Autodesk Inventor part; units mm, degrees
ref_plane "YZ Plane" through (0, 0, 0) normal (1, 0, 0) x (0, 1, 0)
ref_plane "XZ Plane" through (0, 0, 0) normal (0, 1, 0) x (-1, 0, 0)
ref_plane "XY Plane" through (0, 0, 0) normal (0, 0, 1) x (1, 0, 0)
sketch "草圖1" plane through (0, 0, 0) normal (0, 1, 0) x (-1, 0, 0)
  line L0 (14, 14) -> (-14, 14)
  line L1 (-14, 14) -> (-14, -14)
  line L2 (-14, -14) -> (14, -14)
  line L3 (14, -14) -> (14, 14)
  line L4 (14, 14) -> (-14, -14) construction
  line L5 (-14, 14) -> (14, -14) construction
  point P0 (0, 0)
  dimension "d0" = 28
  dimension "d1" = 28
extrude "擠出1" add sketch "草圖1" along normal blind 36
sketch "草圖2" plane through (0, 36, 0) normal (0, 1, 0) x (1, 0, 0)
  circle A0 centre (0, 0) radius 14
extrude "擠出2" add sketch "草圖2" along normal blind 28
sketch "草圖3" plane through (0, 64, 0) normal (0, 1, 0) x (1, 0, 0)
  circle A0 centre (0, 0) radius 8.5
  dimension "d6" = 17
extrude "擠出3" add sketch "草圖3" along normal blind 2
sketch "草圖4" plane through (0, 66, 0) normal (0, 1, 0) x (1, 0, 0)
  circle A0 centre (0, 0) radius 3
  dimension "d9" = 6
extrude "擠出4" add sketch "草圖4" along normal blind 17.5
sketch "草圖5" plane through (0, 83.5, 0) normal (0, 1, 0) x (1, 0, 0)
  circle A0 centre (0, 0) radius 3
  line L0 (-2.5, -1.6583) -> (-2.5, 1.6583)
  point P0 (3, 0)
  dimension "d13" = 5.5
extrude "擠出5" cut sketch "草圖5" against normal blind 15 contours L0 A0 picked at (-2.6056, 0.3442)
sketch "草圖6" plane through (0, 64, 0) normal (0, 1, 0) x (1, 0, 0)
  circle A0 centre (0, 0) radius 11 construction
  line L0 (0, 0) -> (0, 11) construction
  circle A1 centre (0, 0) radius 14
  line L1 (14, 14) -> (0, 14)
  line L2 (-14, -14) -> (0, -14)
  line L3 (14, 14) -> (-14, -14) construction
  circle A2 centre (7.7782, 7.7782) radius 1.5
  circle A3 centre (-7.7782, 7.7782) radius 1.5
  circle A4 centre (-7.7782, -7.7782) radius 1.5
  circle A5 centre (7.7782, -7.7782) radius 1.5
  dimension "d16" = 22
  dimension "d24" = 3
  dimension "d27" = 360
extrude "擠出6" cut sketch "草圖6" against normal blind 10 contours A2 | A3 | A4 | A5
properties part number "28stepper27"
Design review of the part built by this model. Coordinates are the model's own, in mm. A direction names the side the tool comes from. Give positions to 0.01 mm unless a question says otherwise; leave off trailing zeros. Order: outer loops, then holes, each group sorted by start corner. A loop starts at its lowest first (then second) coordinate and runs counter-clockwise, first axis right, second up. Notation, with made-up numbers: (23.25, -4.5) - (51.25, -4.5) arc R12 cw to (51.25, 6.5) - close; hole circle Ø10 at (79.25, 8.25). An arc over 180 degrees is marked (long way). Write item = value, one per line. Start each with the question number.
Q1. We need section A-A on x = 11. State the section outline as (y, z) points.
Q2. To check wall thickness, follow L1, parallel to Y at x = 6.75, z = -1; L2, parallel to Z at x = 8.25, y = 56; L3, parallel to Y at x = 0, z = 12.75. State the ranges of each line that lie inside material, in increasing order. Write a range as from..to.
Q3. Clearance check with flat-ended pins moving along their axes: pin 1 Ø11 at (x, z) = (6, -6.5) entering from +Y; pin 2 Ø1.5 at (x, z) = (-7, -7.5) entering from +Y; pin 3 Ø8 at (x, y) = (7.5, 73) entering from -Z; pin 4 Ø1.5 at (y, z) = (42, -8.5) entering from -X. State where each tip first meets the part, or that it passes through.
Q4. We need section B-B on z = -4.5. State the section outline as (x, y) points, plus the area to 3 significant figures.
Q5. We need section D-D on x = 1.75. State the section outline as (y, z) points, plus the area to 3 significant figures.
Q6. Tool access review of faces 1 (the face through (14, 18, 0)), 2 (the face through (0, 18, 14)), 3 (the face through (-11, 36, 11)), 4 (the face through (-8, 54, 8)), 5 (the face through (-11, 36, -11)): name each direction out of +Z, -Z, +X, -X, +Y, -Y from which nothing blocks a thin tool from reaching the whole face with its end or side.
Q7. Mouldability with a two-part tool opening along Z and no side actions: class faces 6 (the face through (-14, 18, 0)), 7 (the face through (4.57, 64.986, 7.167)), 8 (the face through (8, 54, 8)) as released by +Z, released by -Z, zero draft, split by the parting line, or undercut.
Q8. We need section C-C on y = 71. State the section outline as (x, z) points.
Working result:
q1.outline = (0, -14) - (36, -14) - (36, -8.66) - (64, -8.66) - (64, 8.66) - (36, 8.66) - (36, 14) - (0, 14) - close
q2.L1 = 0..66
q2.L2 = -11.31..-9.2, -6.35..6.35, 9.2..11.31
q2.L3 = 0..64
q3.pin_1 = 66
q3.pin_2 = 64
q3.pin_3 = through
q3.pin_4 = -11.66
q4.outline = (-14, 0) - (14, 0) - (14, 36) - (13.26, 36) - (13.26, 64) - (7.21, 64) - (7.21, 66) - (-7.21, 66) - (-7.21, 64) - (-13.26, 64) - (-13.26, 36) - (-14, 36) - close
q4.area = 1,780 mm²
q5.outline = (0, -14) - (36, -14) - (36, -13.89) - (64, -13.89) - (64, -8.32) - (66, -8.32) - (66, -2.44) - (83.5, -2.44) - (83.5, 2.44) - (66, 2.44) - (66, 8.32) - (64, 8.32) - (64, 13.89) - (36, 13.89) - (36, 14) - (0, 14) - close
q5.area = 1,900 mm²
q6.face_1 = +Z, -Z, +X, +Y, -Y
q6.face_2 = +Z, +X, -X, +Y, -Y
q6.face_3 = +Z, -X, +Y
q6.face_4 = +Y
q6.face_5 = -Z, -X, +Y
q7.face_6 = zero draft
q7.face_7 = split by the parting line
q7.face_8 = undercut
q8.outline = (-2.5, -1.66) arc R3 ccw (long way) to (-2.5, 1.66) - close
